CAD build for the part. Positions are in the model's coordinates, mm. A direction names the side the tool comes from. Round coordinates to 2 decimals unless told otherwise and drop trailing zeros. Loops run counter-clockwise (first coordinate to the right, second up) from the corner with the lowest first, then second, coordinate; pieces in that order, holes last.
from build123d import *

# Parameters (mm, degrees)
SKETCH1_W            = 6.556101186
SKETCH1_H            = 3.6
BOSS_EXTRUDE1_DEPTH  = 2.4
SKETCH2_R            = 0.55
CUT_EXTRUDE1_DEPTH   = 2
LPATTERN1_COUNT      = 8
LPATTERN1_PITCH      = 2.54
LPATTERN1_COUNT_DIR2 = 2
LPATTERN1_PITCH_DIR2 = 7.62


with BuildPart() as part:
    # Sketch1 → Boss-Extrude1 (new body)
    with BuildSketch(Plane(origin=(0, 0, 0), x_dir=(1, 0, 0), z_dir=(0, 1, 0))):
        Polygon((10.14, 2.883247803), (10.14, -2.179313718), (10.14, -5.05), (-10.14, -5.05), (-10.14, -1.8), (-8.64, -1.8), (-8.64, 1.8), (-10.14, 1.8), (-10.14, 5.05), (10.14, 5.05), align=None)
        with Locations((5.031949407, 0)):
            Rectangle(SKETCH1_W, SKETCH1_H, mode=Mode.SUBTRACT)
        with Locations((-3.481949407, 0)):
            Rectangle(SKETCH1_W, SKETCH1_H, mode=Mode.SUBTRACT)
    extrude(amount=BOSS_EXTRUDE1_DEPTH)

    # Sketch2 → Cut-Extrude1 (cut)
    with BuildSketch(Plane(origin=(0, 2.4, 0), x_dir=(1, 0, 0), z_dir=(0, 1, 0))):
        with Locations(Location((-8.89, -3.81, 0), (0, 0, 270))):
            Circle(SKETCH2_R)
    cut_extrude1 = extrude(amount=-CUT_EXTRUDE1_DEPTH, mode=Mode.SUBTRACT)

    # Sketch3 → Revolve1 (revolve)
    with BuildSketch(Plane.XY.offset(3.81), mode=Mode.PRIVATE) as revolve1_sk:
        Polygon((-9.555, 0), (-9.555, -1.9), (-9.15, -1.9), (-9.15, -4.98), (-8.89, -4.98), (-8.89, 0), align=None)
    revolve1 = revolve(revolve1_sk.sketch.rotate(Axis((-8.89, 0, 3.81), (0, 1, 0)), 270), axis=Axis((-8.89, 0, 3.81), (0, 1, 0)))

    # LPattern1: Cut-Extrude1, Revolve1 8 × 2
    with Locations(*[(i * LPATTERN1_PITCH, 0, -j * LPATTERN1_PITCH_DIR2) for i in range(LPATTERN1_COUNT) for j in range(LPATTERN1_COUNT_DIR2) if (i, j) != (0, 0)]):
        add(cut_extrude1, mode=Mode.SUBTRACT)
        add(revolve1)


solid = part.part
Item 1: Mould opens along Z. For faces 4 (the flat face through (10.14, 1, 0)), 5 (the cylindrical face through (3.975, 1.414, 4.335)) say: released by +Z, released by -Z, zero draft, split by the parting line, or undercut.
Verdict:
face 4: zero draft
face 5: undercut
Item 2: Flat gauge pins, fed straight in: P1, Ø4, axis at x = -2.5, y = -3.5, coming from the -Z side; P2, Ø3, axis at x = -5.5, z = -2, coming from the -Y side; P3, Ø1, axis at y = -3, z = -3.5, coming from the +X side. Where does each tip first touch, or does it go through?
Verdict:
P1: stops at z = -4.47
P2: stops at y = -1.9
P3: stops at x = 9.15
Item 3: 3-axis set-ups, long thin cutter, end or side, ignore diameter. For faces 1 (the cylindrical face through (-1.105, 1.414, -3.285)), 2 (the flat face through (-8.64, 1, 0)), 3 (the cylindrical face through (-9.45, -0.96, -4.17)): which of +Z, -Z, +X, -X, +Y, -Y reach the whole face in a straight line?
Verdict:
face 1: +Y
face 2: -X, +Y, -Y
face 3: -Y
Item 4: Cut at B-B (y = -3). State how many separate pieces and enclosed holes the cut face has, plus the area to 3 significant figures.
Verdict:
separate pieces: 16
enclosed holes: 0
area: 3.40 mm2
Item 5: Cut at C-C (z = -0.25). List the corners of the cut face in (x, y).
Verdict:
outline: (-8.64, 0) - (-6.76, 0) - (-6.76, 2.4) - (-8.64, 2.4) - close; (-0.2, 0) - (1.75, 0) - (1.75, 2.4) - (-0.2, 2.4) - close; (8.31, 0) - (10.14, 0) - (10.14, 2.4) - (8.31, 2.4) - close
Item 6: Wall check: L1, parallel to Y at x = -2.25, z = -2; L2, parallel to Y at x = 1, z = 4.25; L3, parallel to Z at x = 0.75, y = -1.75. Give the ranges that are in metal, low to high.
Verdict:
L1: y = 0 to 2.4
L2: y = -1.9 to 0.4
L3: z = -4.22 to -3.4, 3.4 to 4.22
Item 7: Cut at D-D (x = -5.25). List the corners of the cut face in (y, z), plus the area to 3 significant figures.
Verdict:
outline: (0, -5.05) - (2.4, -5.05) - (2.4, -1.8) - (0, -1.8) - close; (0, 1.8) - (2.4, 1.8) - (2.4, 5.05) - (0, 5.05) - close
area: 15.6 mm2
